from build123d import *

# Parameters (mm, degrees)
SKETCH1_R                    = 22.5
BOSS_EXTRUDE1_DEPTH          = 36
SKETCH2_R                    = 11
BOSS_EXTRUDE2_DEPTH          = 3.5
SKETCH5_R                    = 7
CUT_EXTRUDE1_DEPTH           = 3.5
SKETCH6_R                    = 2.5
BOSS_EXTRUDE3_DEPTH          = 22
FILLET1_R                    = 0.5
M2_2X0_45_TAPPED_HOLE1_D     = 1.75
M2_2X0_45_TAPPED_HOLE1_DEPTH = 5.75
M2_2X0_45_TAPPED_HOLE1_TIP   = 0.525753042
SKETCH21_R                   = 2.490055496
BOSS_EXTRUDE6_DEPTH          = 7
F_0_80_TAPPED_HOLE3_D        = 1.19126
F_0_80_TAPPED_HOLE3_DEPTH    = 10
F_0_80_TAPPED_HOLE3_TIP      = 0.357890611
SKETCH17_R                   = 2.5
BOSS_EXTRUDE5_DEPTH          = 6


with BuildPart() as part:
    # Sketch1 → Boss-Extrude1 (new body)
    with BuildSketch(Plane(origin=(0, 0, 0), x_dir=(1, 0, 0), z_dir=(0, 1, 0))):
        Circle(SKETCH1_R)
    extrude(amount=BOSS_EXTRUDE1_DEPTH)

    # Sketch2 → Boss-Extrude2 (add)
    with BuildSketch(Plane(origin=(0, 36, 0), x_dir=(1, 0, 0), z_dir=(0, 1, 0))):
        Circle(SKETCH2_R)
    extrude(amount=BOSS_EXTRUDE2_DEPTH)

    # Sketch5 → Cut-Extrude1 (cut)
    with BuildSketch(Plane(origin=(0, 39.5, 0), x_dir=(1, 0, 0), z_dir=(0, 1, 0))):
        Circle(SKETCH5_R)
    extrude(amount=-CUT_EXTRUDE1_DEPTH, mode=Mode.SUBTRACT)

    # Sketch6 → Boss-Extrude3 (add)
    with BuildSketch(Plane(origin=(0, 36, 0), x_dir=(1, 0, 0), z_dir=(0, 1, 0))):
        Circle(SKETCH6_R)
    extrude(amount=BOSS_EXTRUDE3_DEPTH)

    # Fillet1
    fillet1_edges = [part.edges().sort_by_distance(p)[0] for p in [
        (-2.5, 36, 0),
    ]]
    fillet(fillet1_edges, radius=FILLET1_R)

    # M2.2x0.45 Tapped Hole1
    with Locations(Plane(origin=(-14.276653016, 36, -14.253421631), x_dir=(0, 0, 1), z_dir=(0, 1, 0))):
        with Locations((0, 0), (-0.023231385, 28.530074647), (28.530074647, 0.023231385), (28.506843262, 28.553306032)):
            Hole(M2_2X0_45_TAPPED_HOLE1_D / 2, depth=M2_2X0_45_TAPPED_HOLE1_DEPTH)
            with Locations((0, 0, -(M2_2X0_45_TAPPED_HOLE1_DEPTH + M2_2X0_45_TAPPED_HOLE1_TIP / 2))):  # 118° drill point
                Cone(0, M2_2X0_45_TAPPED_HOLE1_D / 2, M2_2X0_45_TAPPED_HOLE1_TIP, mode=Mode.SUBTRACT)

    # Sketch21 → Boss-Extrude6 (add)
    with BuildSketch(Plane.XZ):
        with Locations((0, -11.5)):
            Circle(SKETCH21_R)
    extrude(amount=BOSS_EXTRUDE6_DEPTH)

    # #0-80 Tapped Hole3
    with Locations(Plane(origin=(-13.163543756, 36, -12.028755501), x_dir=(0, 0, 1), z_dir=(0, 1, 0))):
        with Locations((0, 0), (23.6035957, 26.327087512), (-0.544698362, 27.144135055), (23.875944881, 0.453915302)):
            Hole(F_0_80_TAPPED_HOLE3_D / 2, depth=F_0_80_TAPPED_HOLE3_DEPTH)
            with Locations((0, 0, -(F_0_80_TAPPED_HOLE3_DEPTH + F_0_80_TAPPED_HOLE3_TIP / 2))):  # 118° drill point
                Cone(0, F_0_80_TAPPED_HOLE3_D / 2, F_0_80_TAPPED_HOLE3_TIP, mode=Mode.SUBTRACT)

    # Sketch17 → Boss-Extrude5 (add)
    with BuildSketch(Plane(origin=(0, 0, 0), x_dir=(1, 0, 0), z_dir=(0, 1, 0))):
        with Locations((0, 11.5)):
            Circle(SKETCH17_R)
    extrude(amount=-BOSS_EXTRUDE5_DEPTH)


solid = part.part
Geometry: final body of the model. Coordinates: model frame, mm. A direction names the side the tool comes from. Round coordinates to 2 decimals unless told otherwise and drop trailing zeros. Order: outer loops, then holes, each group sorted by start corner. A loop starts at its lowest first (then second) coordinate and runs counter-clockwise, first axis right, second up. Notation, with made-up numbers: (68.5, -23) -> (86.5, -23) arc R20 cw to (86.5, 14) -> close; hole circle Ø5 at (48, 51.25). An arc over 180 degrees is marked (long way). Put each result on its own line as item: value. Start each with the question number.
Q1. Section D-D on x = 10. Return the cut outline in (y, z).
Q2. Pull-direction query (X, two-part tool) for faces 4 (the cylindrical face through (-0.54, -6.49, -13.93)), 5 (the flat face through (0, -7, -11)), 6 (the flat face through (1, 36, 3)); classes: +X half, -X half, draft (parallel to the pull), parting line (faces both ways), or undercut.
Q3. First-contact query: pin 1 (1.9 mm diameter, centred on x = -13.16, z = -12.03, fed in from +Y); pin 2 (8 mm diameter, centred on x = -1.5, y = 44.5, fed in from +Z); pin 3 (6 mm diameter, centred on x = 7.5, y = 49, fed in from +Z); pin 4 (1.1 mm diameter, centred on x = -12.71, z = 11.85, fed in from +Y). Flat tips, straight axial feed; report the tip coordinate or a pass-through.
Q4. Section C-C on y = 46. Return the cut outline in (x, z).
Q5. Section A-A on z = 0. Return the cut outline in (x, y).
Q6. Line query: probe 1 along X at (y, z) = (37.5, 0); probe 2 along Y at (x, z) = (9, 15); probe 3 along Y at (x, z) = (3, 10.5). Output: solid intervals per line, ascending.
Q7. Reachability of faces 1 (the cylindrical face through (13.477, 33.085, -14.68)), 2 (the cylindrical face through (-0.54, -2.96, -9.06)), 3 (the cylindrical face through (10.382, 17.748, 19.961)) from +Z, -Z, +X, -X, +Y, -Y: full face, straight path, thin tool, end or side. Return the list, or none.
Ans:
1. outline: (0, -20.16) -> (36, -20.16) -> (36, -4.58) -> (39.5, -4.58) -> (39.5, 4.58) -> (36, 4.58) -> (36, 20.16) -> (0, 20.16) -> close
2. face 4: parting line
2. face 5: draft
2. face 6: undercut
3. pin 1: stops at y = 36
3. pin 2: stops at z = 2.5
3. pin 3: passes through
3. pin 4: stops at y = 25.97
4. outline: circle Ø5 at (0, 0)
5. outline: (-22.5, 0) -> (22.5, 0) -> (22.5, 36) -> (11, 36) -> (11, 39.5) -> (7, 39.5) -> (7, 36) -> (3, 36) arc R0.5 cw to (2.5, 36.5) -> (2.5, 58) -> (-2.5, 58) -> (-2.5, 36.5) arc R0.5 cw to (-3, 36) -> (-7, 36) -> (-7, 39.5) -> (-11, 39.5) -> (-11, 36) -> (-22.5, 36) -> close
6. probe 1: x = -11 to -7, -2.5 to 2.5, 7 to 11
6. probe 2: y = 0 to 36
6. probe 3: y = 0 to 39.5
7. face 1: +Y
7. face 2: -Y
7. face 3: +Y, -Y
